Could you check a few things on this model? Use its own coordinates, in mm. Give positions to 0.01 mm unless a question says otherwise; leave off trailing zeros. Order: outer loops, then holes, each group sorted by start corner. A loop starts at its lowest first (then second) coordinate and runs counter-clockwise, first axis right, second up. Notation, with made-up numbers: (-22.75, 85.25) -> (2.25, 85.25) arc R28 ccw to (2.25, 109.25) -> close; hole circle Ø8 at (9.5, 15.25). An arc over 180 degrees is marked (long way). Write each question's results on one line, items separated by ' | '.
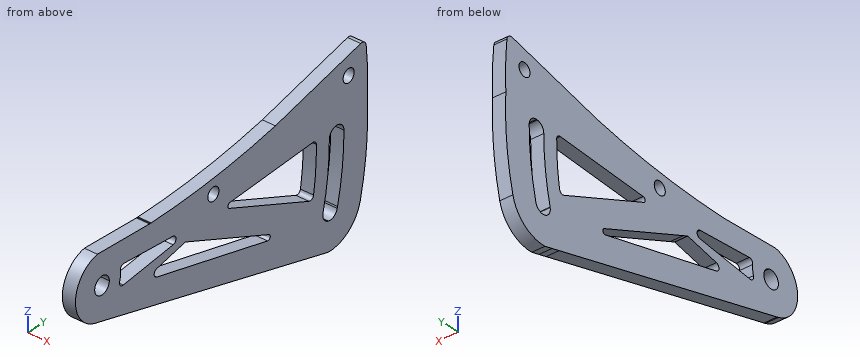
```python
from build123d import *

# Parameters (mm, degrees)
F0_R     = 2.5
F1_DEPTH = 5


with BuildPart() as f1:
    # F0 (on Right) → F1 (new body)
    with BuildSketch(Plane.YZ):
        with BuildLine():
            ThreePointArc((102.1820204733, -38.7985140437), (111.3688992979, -36.087326884), (116.6625133499, -28.1044120891))
            ThreePointArc((116.6625133499, -28.1044120891), (119.4793240413, -11.1665181072), (119.8499061326, 6))
            ThreePointArc((119.8499061326, 6), (119.9551556627, 15.2803399129), (119.3428752162, 24.5410579746))
            ThreePointArc((119.3428752162, 24.5410579746), (118.5020303548, 25.9696085801), (116.872434029, 26.2732411356))
            Line((116.872434029, 26.2732411356), (78.344444671, 16.7187866332))
            ThreePointArc((78.344444671, 16.7187866332), (50.4120849121, 12.3407543123), (22.1844688263, 10.7327808001))
            ThreePointArc((22.1844688263, 10.7327808001), (22.0736743793, 10.7245163933), (21.9626931438, 10.7193322557))
            ThreePointArc((21.9626931438, 10.7193322557), (21.897134346, 10.7177196915), (21.8315579223, 10.717182122))
            ThreePointArc((21.8315579223, 10.717182122), (21.6468606164, 10.7214485341), (21.4625573078, 10.7342386694))
            Line((21.4625573078, 10.7342386694), (-2.0614712889, 11.8216046341))
            ThreePointArc((-2.0614712889, 11.8216046341), (-11.9825923491, 0.6461273838), (-3.3207151947, -11.5313854586))
            Line((-3.3207151947, -11.5313854586), (-2.6824780436, -11.696337527))
            Line((-2.6824780436, -11.696337527), (95.7506312441, -37.1363247556))
            Line((95.7506312441, -37.1363247556), (98.966975845, -37.9675873883))
            Line((98.966975845, -37.9675873883), (102.1820204733, -38.7985140437))
        make_face()
        with BuildLine():
            Line((74.7801037599, -21.3838166757), (24.7079464878, -9.2750381753))
            ThreePointArc((24.7079464878, -9.2750381753), (23.5605944603, -7.8024693416), (24.7363828951, -6.3525047896))
            Line((24.7363828951, -6.3525047896), (37.64646566, -3.4952066638))
            Line((37.64646566, -3.4952066638), (39.6840657747, -4.3584005208))
            Line((39.6840657747, -4.3584005208), (75.4052290095, -19.4910501744))
            ThreePointArc((75.4052290095, -19.4910501744), (75.9647072114, -20.7254429281), (74.7801037599, -21.3838166757))
        make_face(mode=Mode.SUBTRACT)
        with BuildLine():
            ThreePointArc((96.8537245562, 1.1511288497), (96.5833908806, -7.3224083499), (95.5731457656, -15.7398496344))
            ThreePointArc((95.5731457656, -15.7398496344), (94.8167325655, -16.8099987725), (93.5079720679, -16.8772748216))
            Line((93.5079720679, -16.8772748216), (57.4962823848, -1.6215486902))
            ThreePointArc((57.4962823848, -1.6215486902), (56.9006424726, -0.5323364967), (57.8241552759, 0.297298489))
            Line((57.8241552759, 0.297298489), (95.2605289234, 2.6303977234))
            ThreePointArc((95.2605289234, 2.6303977234), (96.3744600577, 2.2325362159), (96.8537245562, 1.1511288497))
        make_face(mode=Mode.SUBTRACT)
        with BuildLine():
            ThreePointArc((106.0047579916, 3.2999965699), (108.335133976, 2.3317695671), (109.3, 0))
            ThreePointArc((109.3, 0), (108.5733985389, -12.5820161229), (106.403254717, -24.9967475011))
            ThreePointArc((106.403254717, -24.9967475011), (106.3321059009, -25.2976926752), (106.2601059096, -25.5984353445))
            ThreePointArc((106.2601059096, -25.5984353445), (104.7727098756, -27.6413708088), (102.2762174538, -28.0331077884))
            ThreePointArc((102.2762174538, -28.0331077884), (102.0809432414, -27.9794930887), (101.8893251401, -27.9140021941))
            ThreePointArc((101.8893251401, -27.9140021941), (100.1771054463, -26.4459442797), (99.8077413449, -24.2209812507))
            ThreePointArc((99.8077413449, -24.2209812507), (99.8054980044, -24.2204076148), (99.803254717, -24.2198337711))
            ThreePointArc((99.803254717, -24.2198337711), (99.8234961781, -24.1362716836), (99.8436676753, -24.0526926796))
            ThreePointArc((99.8436676753, -24.0526926796), (101.9834169614, -12.1108490566), (102.7, 0))
            ThreePointArc((102.7, 0), (103.5243491823, 2.1820066519), (105.5855472903, 3.2738706376))
            ThreePointArc((105.5855472903, 3.2738706376), (105.7947365556, 3.2936100131), (106.0047579916, 3.2999965699))
        make_face(mode=Mode.SUBTRACT)
        with BuildLine():
            ThreePointArc((0.9709435511, 3.1539290767), (2.6546293261, 1.960342608), (3.3, 0))
            ThreePointArc((3.3, 0), (-2.6546293261, -1.960342608), (0.9709435511, 3.1539290767))
        make_face(mode=Mode.SUBTRACT)
        with BuildLine():
            ThreePointArc((9.5663779465, -4.5835158726), (8.220643901, -4.0486256327), (7.9543036044, -2.6251894605))
            ThreePointArc((7.9543036044, -2.6251894605), (8.3387505543, -0.792341295), (8.3063784002, 1.0801126827))
            ThreePointArc((8.3063784002, 1.0801126827), (8.7016404445, 2.3016729085), (9.8971035196, 2.769977836))
            Line((9.8971035196, 2.769977836), (32.0235012294, 1.2433501427))
            ThreePointArc((32.0235012294, 1.2433501427), (33.4196537084, -0.210693525), (32.1078987642, -1.7413089889))
            Line((32.1078987642, -1.7413089889), (9.5663779465, -4.5835158726))
        make_face(mode=Mode.SUBTRACT)
        with Locations((50.3031872213, 6.8563437089)):
            Circle(F0_R, mode=Mode.SUBTRACT)
        with Locations((111.4225909114, 17.8264938295)):
            Circle(F0_R, mode=Mode.SUBTRACT)
        with BuildLine():
            ThreePointArc((-3.3207151947, -11.5313854586), (-3.0027295184, -11.618244938), (-2.6824780436, -11.696337527))
            Line((-2.6824780436, -11.696337527), (-3.3207151947, -11.5313854586))
        make_face()
        with BuildLine():
            ThreePointArc((21.9626931438, 10.7193322557), (22.0736743793, 10.7245163933), (22.1844688263, 10.7327808001))
            ThreePointArc((22.1844688263, 10.7327808001), (22.0739250085, 10.7319598925), (21.9633808826, 10.731181571))
            ThreePointArc((21.9633808826, 10.731181571), (21.9630378123, 10.7252568669), (21.9626931438, 10.7193322557))
        make_face()
        with BuildLine():
            ThreePointArc((21.8315579223, 10.717182122), (21.897134346, 10.7177196915), (21.9626931438, 10.7193322557))
            ThreePointArc((21.9626931438, 10.7193322557), (21.9630378123, 10.7252568669), (21.9633808826, 10.731181571))
            ThreePointArc((21.9633808826, 10.731181571), (21.7716697335, 10.7299327404), (21.5799577929, 10.728811993))
            Line((21.5799577929, 10.728811993), (21.8315579223, 10.717182122))
        make_face()
        with BuildLine():
            ThreePointArc((21.4625573078, 10.7342386694), (21.6468606164, 10.7214485341), (21.8315579223, 10.717182122))
            Line((21.8315579223, 10.717182122), (21.5799577929, 10.728811993))
            Line((21.5799577929, 10.728811993), (21.4625573078, 10.7342386694))
        make_face()
    extrude(amount=F1_DEPTH)


solid = f1.part
```
Q1. Suppose I cut it at C-C on y = 51.5. Please give me the cut outline in (x, z), and give its area (3 significant figures).
Here are the results:
outline: (0, -25.7) -> (5, -25.7) -> (5, -15.75) -> (0, -15.75) -> close; (0, -9.36) -> (5, -9.36) -> (5, 4.66) -> (0, 4.66) -> close; (0, 9.05) -> (5, 9.05) -> (5, 12.46) -> (0, 12.46) -> close | area: 137 mm²
Q2. Suppose I cut it at B-B on x = 1.35. State how many separate pieces and enclosed holes the cut face has, and give its area (3 significant figures).
Here are the results:
separate pieces: 1 | enclosed holes: 7 | area: 4,170 mm²
Q3. Suppose I cut it at A-A on y = 30. Please give me the cut outline in (x, z), and give its area (3 significant figures).
Here are the results:
outline: (0, -20.14) -> (5, -20.14) -> (5, -10.55) -> (0, -10.55) -> close; (0, -5.19) -> (5, -5.19) -> (5, -2.01) -> (0, -2.01) -> close; (0, 1.38) -> (5, 1.38) -> (5, 10.9) -> (0, 10.9) -> close | area: 111 mm²
Q4. Suppose I cut it at D-D on z = -30. Please give me the cut outline in (x, y), and give its area (3 significant figures).
Here are the results:
outline: (0, 68.14) -> (5, 68.14) -> (5, 116.06) -> (0, 116.06) -> close | area: 240 mm²
Q5. I need wall thicknesses on line 1 along Z through (x, y) = (0.65, 67); line 2 along Z through (x, y) = (4.85, 57.5); line 3 along Y through (x, z) = (4.35, 3). Which ranges of each line are inside material? Lowest first, please.
Here are the results:
line 1: z = -29.71 to -19.5, -15.93 to -5.65, 0.87 to 14.6 | line 2: z = -27.25 to -17.21, -11.91 to -1.62, 0.22 to 13.19 | line 3: y = -11.62 to -1.37, 1.37 to 104.63, 107.37 to 119.96
Q6. I'm going to push flat-ended pins straight in: pin 1 Ø1 at (y, z) = (93, -15) entering from -X; pin 2 Ø3 at (x, y) = (3.5, 45) entering from +Z. Where does each tip first touch, or does it pass through?
Here are the results:
pin 1: passes through | pin 2: stops at z = 11.95
